The listing builds one solid part. Answer for the finished solid, in the listing's coordinates (mm). Face numbers are marked on the shaded views. A direction names the side the tool comes from. Give positions to 0.01 mm unless a question says otherwise; leave off trailing zeros. Order: outer loops, then holes, each group sorted by start corner. A loop starts at its lowest first (then second) coordinate and runs counter-clockwise, first axis right, second up. Notation, with made-up numbers: (-23.5, 33.25) -> (-0.5, 33.25) arc R23 ccw to (-0.5, 51.25) -> close; hole circle Ø2 at (-10, 45). An arc over 180 degrees is marked (long way). Answer as a JSON object with one key per item and string values. Group by question number.
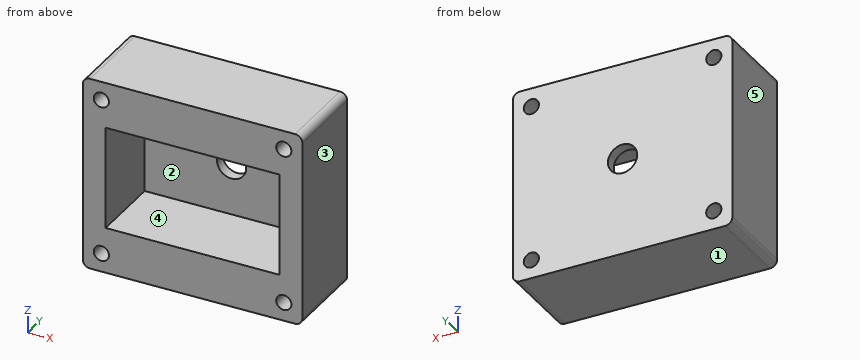
```python
from build123d import *

# Parameters (mm, degrees)
F0_W     = 60
F0_H     = 53
F1_DEPTH = 23
F2_W     = 47.5
F2_H     = 28
F3_DEPTH = 20
F4_R     = 2
F5_R     = 2
F6_R     = 4
F7_DEPTH = 3
F8_R     = 2.075
F9_DEPTH = 23


with BuildPart() as f1:
    # F0 (on Front) → F1 (new body)
    with BuildSketch(Plane.XZ):
        Rectangle(F0_W, F0_H)
    extrude(amount=F1_DEPTH)

    # F2 (on face) → F3 (cut)
    with BuildSketch(Plane.XZ.offset(23)):
        Rectangle(F2_W, F2_H)
    extrude(amount=-F3_DEPTH, mode=Mode.SUBTRACT)

    # F4
    f4_edges = [f1.edges().sort_by_distance(p)[0] for p in [
        (-30, -11.5, -26.5),
    ]]
    fillet(f4_edges, radius=F4_R)

    # F5
    f5_edges = [f1.edges().sort_by_distance(p)[0] for p in [
        (30, -11.5, -26.5),
        (30, -11.5, 26.5),
        (-30, -11.5, 26.5),
    ]]
    fillet(f5_edges, radius=F5_R)

    # F6 (on face) → F7 (cut)
    with BuildSketch(Plane(origin=(0, 0, 0), x_dir=(-1, 0, 0), z_dir=(0, 1, 0))):
        Circle(F6_R)
    extrude(amount=-F7_DEPTH, mode=Mode.SUBTRACT)

    # F8 (on face) → F9 (cut)
    with BuildSketch(Plane.XZ.offset(23)):
        with Locations((-24.925, 21.425)):
            Circle(F8_R)
        with Locations((24.925, 21.425)):
            Circle(F8_R)
        with Locations((24.925, -21.425)):
            Circle(F8_R)
        with Locations((-24.925, -21.425)):
            Circle(F8_R)
    extrude(amount=-F9_DEPTH, mode=Mode.SUBTRACT)


solid = f1.part
```
(1) Find the intervals of material crossed by line 1 along Z through (x, y) = (3, -12); line 2 along Z through (x, y) = (24, -4); line 3 along X through (y, z) = (-6, 3), in increasing order. Write a range as [from, to].
(2) A cutting plane is placed at C-C (z = 9.5). Determine the outline of the cut face in (x, y).
(3) A cutting plane is placed at B-B (z = 0). Determine the outline of the cut face in (x, y).
(4) A cutting plane is placed at D-D (y = -5.5). Determine the outline of the cut face in (x, z) (3 decimals), and give its area (3 significant figures).
(5) Flat-ended cylindrical pins translate along their axes: pin 1 Ø2 at (x, z) = (7.5, -4) entering from -Y; pin 2 Ø7 at (x, z) = (0, 0) entering from +Y. Find the tip coordinate at first contact, or state that the pin passes through.
(6) Which of the six approach directions +Z, -Z, +X, -X, +Y, -Y give full straight-line access (tool end or side, diameter ignored) to the marked faces 1 and 2?
(7) A cutting plane is placed at A-A (x = 0). Determine the outline of the cut face in (y, z).
(8) For a pull along X with two mould halves and no side action, classify the marked faces 3, 4 and 5 as +X half, -X half, draft (parallel to the pull), parting line (faces both ways), or undercut.
Check sheet entries:
{
 "1": {"line 1": "z = [-26.5, -14], [14, 26.5]", "line 2": "z = [-26.5, -23.28], [-19.57, 19.57], [23.28, 26.5]", "line 3": "x = [-30, -23.75], [23.75, 30]"},
 "2": {"outline": "(-30, -23) -> (-23.75, -23) -> (-23.75, -3) -> (23.75, -3) -> (23.75, -23) -> (30, -23) -> (30, 0) -> (-30, 0) -> close"},
 "3": {"outline": "(-30, -23) -> (-23.75, -23) -> (-23.75, -3) -> (-4, -3) -> (-4, 0) -> (-30, 0) -> close; (4, -3) -> (23.75, -3) -> (23.75, -23) -> (30, -23) -> (30, 0) -> (4, 0) -> close"},
 "4": {"outline": "(-30, -24.5) arc R2 ccw to (-28, -26.5) -> (28, -26.5) arc R2 ccw to (30, -24.5) -> (30, 24.5) arc R2 ccw to (28, 26.5) -> (-28, 26.5) arc R2 ccw to (-30, 24.5) -> close; hole circle Ø4.15 at (-24.925, -21.425); hole circle Ø4.15 at (-24.925, 21.425); hole (-23.75, -14) -> (23.75, -14) -> (23.75, 14) -> (-23.75, 14) -> close; hole circle Ø4.15 at (24.925, -21.425); hole circle Ø4.15 at (24.925, 21.425)", "area": "1,790 mm2"},
 "5": {"pin 1": "stops at y = -3", "pin 2": "passes through"},
 "6": {"face 1": "-Z, +X, -X, +Y, -Y", "face 2": "-Y"},
 "7": {"outline": "(-23, -26.5) -> (0, -26.5) -> (0, -4) -> (-3, -4) -> (-3, -14) -> (-23, -14) -> close; (-23, 14) -> (-3, 14) -> (-3, 4) -> (0, 4) -> (0, 26.5) -> (-23, 26.5) -> close"},
 "8": {"face 3": "+X half", "face 4": "undercut", "face 5": "-X half"}
}
